from build123d import *

# Parameters (mm, degrees)
F3_DEPTH  = 25.4
F4_W      = 12.7
F4_H      = 7.9375
F5_DEPTH  = 25.4
F6_SIZE   = 2.54
F7_R      = 9.525
F8_DEPTH  = 25.4
F9_SIZE   = 1.27
F10_R     = 3.96875
F11_DEPTH = 25.4


with BuildPart() as f1:
    # F0 (on Top) → F1 (revolve)
    with BuildSketch(Plane.XY):
        Polygon((-12.7, 8.3694059759), (-10.541, 2.1945910865), (-10.541, -4.3305940241), (-8.001, -4.3305940241), (-8.001, 0), (-6.858, 0), (-6.858, 9.144), (-6.096, 9.144), (-6.096, 11.684), (-10.16, 14.030351494), (-10.16, 24.190351494), (-6.096, 26.536702988), (-6.096, 29.076702988), (-10.16, 31.423054482), (-10.16, 41.583054482), (-6.096, 43.9294059759), (-6.096, 46.4694059759), (-12.7, 46.4694059759), align=None)
    revolve(axis=Axis((0, 65.4240736527, 0), (0, 1, 0)))

    # F2 (on face) → F3 (cut)
    with BuildSketch(Plane(origin=(0, 46.4694059759, 0), x_dir=(-1, 0, 0), z_dir=(0, 1, 0))):
        Polygon((-25.4, 8.636), (0, 8.636), (25.4, 8.636), (25.4, 25.7254446054), (-25.4, 25.7254446054), align=None)
    extrude(amount=-F3_DEPTH, mode=Mode.SUBTRACT)

    # F4 (on face) → F5 (cut)
    with BuildSketch(Plane(origin=(0, 46.4694059759, 0), x_dir=(-1, 0, 0), z_dir=(0, 1, 0))):
        Polygon((-8.001, 0), (-8.001, 3.96875), (-20.701, 3.96875), (-20.701, -3.96875), (-8.001, -3.96875), align=None)
        with Locations((14.351, 0)):
            Rectangle(F4_W, F4_H)
    extrude(amount=-F5_DEPTH, mode=Mode.SUBTRACT)

    # F6
    f6_edges = [f1.edges().sort_by_distance(p)[0] for p in [
        (10.939674, 46.469406, 6.450855),
        (0, 46.469406, -12.7),
        (-10.939674, 46.469406, 6.450855),
    ]]
    chamfer(f6_edges, length=F6_SIZE)

    # F7 (on face) → F8 (cut)
    with BuildSketch(Plane.XY.offset(8.636)):
        with Locations((0, 23.0734321734)):
            Circle(F7_R)
    extrude(amount=F8_DEPTH, mode=Mode.SUBTRACT)

    # F9
    f9_edges = [f1.edges().sort_by_distance(p)[0] for p in [
        (10.541, -4.330594, 0),
    ]]
    chamfer(f9_edges, length=F9_SIZE)

    # F10 (on face) → F11 (cut, symmetric)
    with BuildSketch(Plane.YZ.offset(8.001)):
        with Locations((21.0694059759, 0)):
            Circle(F10_R)
    extrude(amount=F11_DEPTH, both=True, mode=Mode.SUBTRACT)


solid = f1.part
Build history of the part. All positions in model axes, mm. A direction names the side the tool comes from. Give positions to 0.01 mm unless a question says otherwise; leave off trailing zeros. Order: outer loops, then holes, each group sorted by start corner. A loop starts at its lowest first (then second) coordinate and runs counter-clockwise, first axis right, second up. Notation, with made-up numbers: M 87.25,-25 L 126.25,-25 A13 cw 126.25,-10 Z; hole C 48,48.5 d9. An arc over 180 degrees is marked long. Put each result on its own line as item: value.
Item 1: Which spindle directions (+Z, -Z, +X, -X, +Y, -Y) get a long thin tool onto all of the face, cutting with end or side? Do faces 4 (the face through (10, 34, 3.969)), 5 (the face through (-10, 34, 3.969)), 6 (the face through (0.17, 36.57, -10.16)). Say none if no direction does.
Results are:
face 4: +X, +Y
face 5: -X, +Y
face 6: none
Item 2: Cut at A-A on y = 22. Write the cut outline in (x, z).
Results are:
outline: M -12.06,-3.97 A12.7 ccw 12.06,-3.97 L 9.35,-3.97 A10.16 cw -9.35,-3.97 Z; M -12.06,3.97 L -9.35,3.97 A10.16 cw -5.35,8.64 L -9.31,8.64 A12.7 ccw Z; M 5.35,8.64 A10.16 cw 9.35,3.97 L 12.06,3.97 A12.7 ccw 9.31,8.64 Z
Item 3: Drop flat-ended pins along their axis: pin 1 Ø3.5 at (x, y) = (-11, 30) entering from +Z; pin 2 Ø14.5 at (x, z) = (0, 0) entering from +Y; pin 3 Ø8 at (x, z) = (-2.5, -2) entering from -Y; pin 4 Ø1 at (y, z) = (28, 3.5) entering from +X. Give the stop position or say it passes through.
Results are:
pin 1: z = 8.64
pin 2: y = 46.47
pin 3: y = 0
pin 4: x = 12.06
Item 4: Wall check: probe 1 along Y at (x, z) = (-6.5, -3); probe 2 along Y at (x, z) = (-3, -8); probe 3 along X at (y, z) = (19.5, -7.5). Give the ranges that are in metal, low to high.
Results are:
probe 1: 0 to 12.3, 25.92 to 29.69, 43.32 to 46.47
probe 2: -4.33 to 13.1, 25.12 to 30.49, 42.52 to 46.47
probe 3: -10.25 to -6.85, 6.85 to 10.25
Item 5: Cut at D-D on y = 3. Write the cut outline in (x, z), then the cut area to 3 significant figures.
Results are:
outline: C 0,0 d21.65; hole C 0,0 d13.72
area: 220 mm2
Item 6: Pull direction Z, two halves, no side cores. Call faces 1 (the face through (0.794, 45.217, 6.044)), 2 (the face through (0, 28, 8.636)), 3 (the face through (0.18, 46.35, -10.28)): +Z half, -Z half, draft (parallel to the pull), parting line (faces both ways), or undercut.
Results are:
face 1: undercut
face 2: +Z half
face 3: -Z half
Item 7: Cut at B-B on z = 2. Count the separate pieces of the cut face and the enclosed holes in it, then the cut area to 3 significant figures.
Results are:
separate pieces: 6
enclosed holes: 0
area: 213 mm2
